Part model, mm, in its own coordinate system. A direction names the side the tool comes from. Coordinates: 2 decimals unless noted, no trailing zeros. Order: outer loops, then holes, each group sorted by start corner. A loop starts at its lowest first (then second) coordinate and runs counter-clockwise, first axis right, second up.
from build123d import *

# Parameters (mm, degrees)
CUT_EXTRUDE_1_DEPTH      = 10
PATTERN_CIRCULAR_1_COUNT = 4
SKETCH_3_R               = 3
SKETCH_3_R_2             = 1.5
CUT_EXTRUDE_2_DEPTH      = 5


with BuildPart() as part:
    # Sketch 1 → Revolve 2 (revolve)
    with BuildSketch(Plane(origin=(0, 0, 0), x_dir=(0, 0, -1), z_dir=(1, 0, 0))):
        Polygon((13.999479922, 22.7), (12.5, 24.2), (4.5, 24.2), (4.5, 26.2), (2.5, 26.2), (2.5, 36.2), (0, 36.2), (0, 23.2), (11.5, 23.2), (11.999479922, 22.2), (11.999479922, 20), (12.999479922, 20), (12.999479922, 4), (4.249479922, 4), (4.249479922, 3), (0, 3), (0, 0), (0.75, 0), (0.75, 0.540825023), (1.5, 0.540825023), (1.5, 0.2), (12, 0.2), (14, 1.8), (14, 2.8), (10, 2.8), (10, 3), (13.999479922, 3), (13.999479922, 21), (12.499479922, 21), (12.499479922, 21.2), (13.999479922, 21.2), align=None)
    revolve(axis=Axis((0, 0, 0), (0, 1, 0)))

    # Sketch 2 → Cut-Extrude 1 (cut)
    with BuildSketch(Plane(origin=(0, 24.2, 0), x_dir=(1, 0, 0), z_dir=(0, 1, 0))):
        with BuildLine():
            Line((-2, 12.338962679), (-2, 8.338962679))
            ThreePointArc((-2, 8.338962679), (0, 6.338962679), (2, 8.338962679))
            Line((2, 8.338962679), (2, 12.338962679))
            ThreePointArc((2, 12.338962679), (0, 12.5), (-2, 12.338962679))
        make_face()
        with BuildLine():
            Line((-5.282728272, 11.328847338), (-1.690473047, 3.625231148))
            ThreePointArc((-1.690473047, 3.625231148), (-2.032137638, 2.032137638), (-3.625231148, 1.690473047))
            Line((-3.625231148, 1.690473047), (-11.328847338, 5.282728272))
            ThreePointArc((-11.328847338, 5.282728272), (-8.838834765, 8.838834765), (-5.282728272, 11.328847338))
        make_face()
    cut_extrude_1 = extrude(amount=-CUT_EXTRUDE_1_DEPTH, mode=Mode.SUBTRACT)

    # Pattern Circular 1: Cut-Extrude 1 ×4 about axis
    pattern_circular_1_axis = Axis((0, 0, 0), (0, 1, 0))
    for i in range(1, PATTERN_CIRCULAR_1_COUNT):
        add(cut_extrude_1.rotate(pattern_circular_1_axis, i * 360 / PATTERN_CIRCULAR_1_COUNT), mode=Mode.SUBTRACT)

    # Sketch 3 → Cut-Extrude 2 (cut)
    with BuildSketch(Plane.XZ.offset(-0.2)):
        with Locations((8, 0)):
            Circle(SKETCH_3_R)
        with Locations((0, 8)):
            Circle(SKETCH_3_R)
        with Locations((-8, 0)):
            Circle(SKETCH_3_R)
        with Locations((0, -8)):
            Circle(SKETCH_3_R)
        with Locations((6.333333333, 7.080881929)):
            Circle(SKETCH_3_R_2)
        with Locations((-6.333333333, -7.080881929)):
            Circle(SKETCH_3_R_2)
        with Locations((-5.96284794, 5.333333333)):
            Circle(SKETCH_3_R_2)
        with Locations((5.96284794, -5.333333333)):
            Circle(SKETCH_3_R_2)
    extrude(amount=-CUT_EXTRUDE_2_DEPTH, mode=Mode.SUBTRACT)


solid = part.part
Q1. Which spindle directions (+Z, -Z, +X, -X, +Y, -Y) get a long thin tool onto all of the face, cutting with end or side? Do faces 5 (the face through (-4, 20, -12)), 6 (the face through (8.8, 22.72, -8.88)), 7 (the face through (5, 2, 0)). Say none if no direction does.
Results list:
face 5: none
face 6: +Y
face 7: -Y
Q2. Cut at A-A on y = 11.5. Write the cut outline in (x, z).
Results list:
outline: circle Ø28 at (0, 0); hole circle Ø26 at (0, 0)
Q3. Cut at B-B on x = 0. Count the separate pieces of the cut face and the enclosed holes in it, and give its area (3 significant figures).
Results list:
separate pieces: 8
enclosed holes: 0
area: 170 mm2
Q4. Mould opens along Y. For faces 1 (the face through (3.516, 22.693, -11.215)), 2 (the face through (2, 23.4, 10.6)), 3 (the face through (2, 26.2, -2)), 4 (the face through (0, 0.541, -1)) say: pulls with the +Y half, pulls with the -Y half, needs draft (parallel to the pull), parting line crosses it, or undercut.
Results list:
face 1: undercut
face 2: needs draft
face 3: pulls with the +Y half
face 4: pulls with the -Y half
Q5. Pin check, flat tips, straight feed: pin 1 Ø6.5 at (x, z) = (2, -10) entering from +Y; pin 2 Ø5 at (x, y) = (6, 14) entering from +Z; pin 3 Ø12 at (y, z) = (12.5, 4) entering from +X; pin 4 Ø1.5 at (y, z) = (32, 4.5) entering from +X. Stop position of each tip, or through.
Results list:
pin 1: stops at y = 24.2
pin 2: stops at z = 13.55
pin 3: stops at x = 14
pin 4: passes through
Q6. Wall check: line 1 along Z through (x, y) = (0.5, 6); line 2 along Y through (x, z) = (1.25, 13.25); line 3 along X through (y, z) = (24, -7.75). Give the ranges that are in metal, low to high.
Results list:
line 1: z = -13.99 to -12.99, 12.99 to 13.99
line 2: y = 1.25 to 2.8, 3 to 21, 21.2 to 23.39
line 3: x = -10.06 to -9.81, -3.61 to -1.91, 1.91 to 3.61, 9.81 to 10.06
Q7. Cut at C-C on y = 25. Write the cut outline in (x, z).
Results list:
outline: circle Ø9 at (0, 0)
